Verification items for the finished model (mm, model axes). A direction names the side the tool comes from. Coordinates: 2 decimals unless noted, no trailing zeros. Write each loop counter-clockwise with the first axis right and the second up, starting at its lowest first coordinate (ties: lowest second). Pieces come first, ordered by that corner, then holes. Notation, with made-up numbers: M -17.5,-12.5 L 1.5,-12.5 A15 ccw 1.5,15.5 Z; hole C 1.25,30 d9. An arc over 180 degrees is marked long. Answer in a Markdown table with one row per item.
from build123d import *

# Parameters (mm, degrees)
PAD004_DEPTH    = 29
POCKET001_DEPTH = 5
POCKET002_DEPTH = 5
SKETCH008_R     = 5
POCKET003_DEPTH = 10
SKETCH015_R     = 2
POCKET007_DEPTH = 24.001


with BuildPart() as obj1:
    # Sketch004 → Pad004 (new body)
    with BuildSketch(Plane.XY):
        with BuildLine():
            Line((0, 40), (0, 0))
            Line((0, 0), (160, 0))
            Line((160, 15), (160, 0))
            Line((125, 15), (160, 15))
            ThreePointArc((115, 25), (117.928932, 17.928932), (125, 15))
            Line((115, 42.094566), (115, 25))
            Line((90, 42.094566), (115, 42.094566))
            Line((90, 42.094566), (90, 20))
            ThreePointArc((80, 10), (87.071068, 12.928932), (90, 20))
            Line((30, 10), (80, 10))
            ThreePointArc((10, 30), (15.857864, 15.857864), (30, 10))
            Line((10, 40), (10, 30))
            Line((0, 40), (10, 40))
        make_face()
    extrude(amount=PAD004_DEPTH)

    # Sketch006 (on Face15 of Pad004) → Pocket001 (cut)
    with BuildSketch(Plane.XY.offset(29)):
        Polygon((5, 45), (5, 5), (100, 5), (100, -8.029739), (275.374889, -8.029739), (275.374889, 45), align=None)
    extrude(amount=-POCKET001_DEPTH, mode=Mode.SUBTRACT)

    # Sketch007 (on Face2 of Pocket001) → Pocket002 (cut)
    with BuildSketch(Plane(origin=(0, 0, 0), x_dir=(1, 0, 0), z_dir=(0, 0, -1))):
        Polygon((5, -5), (5, -45), (160, -45), (160, 8.546066), (45, 8.546066), (45, -5), align=None)
    extrude(amount=-POCKET002_DEPTH, mode=Mode.SUBTRACT)

    # Sketch008 (on Face4 of Pocket002) → Pocket003 (cut)
    with BuildSketch(Plane.XY.offset(24)):
        with Locations((110, 10)):
            Circle(SKETCH008_R)
    extrude(amount=-POCKET003_DEPTH, mode=Mode.SUBTRACT)

    # Sketch015 (on Face4 of Pocket003) → Pocket007 (cut, through all)
    with BuildSketch(Plane.XY.offset(24)):
        with Locations((11, 11)):
            Circle(SKETCH015_R)
        with Locations((94, 11)):
            Circle(SKETCH015_R)
        with Locations((94, 36)):
            Circle(SKETCH015_R)
        with Locations((106, 36)):
            Circle(SKETCH015_R)
        with Locations((124, 6)):
            Circle(SKETCH015_R)
        with Locations((154, 6)):
            Circle(SKETCH015_R)
    extrude(amount=-POCKET007_DEPTH, mode=Mode.SUBTRACT)


with BuildPart() as obj1_1:
    # Body004 placement: moved
    add(obj1.part.moved(Location((-250, -150, 0))))


with BuildPart() as obj2:
    # Part__Mirroring001: instance of obj1
    add(obj1_1.part.mirror(Plane(origin=(0, 0, 0), x_dir=(0, -1, 0), z_dir=(1, 0, 0))))


solid = obj2.part
1) Tool access check on faces 1 (the face through (225, -145, 2)), 2 (the face through (234.297, -133.986, 14.367)), 3 (the face through (108, -135, 14)), 4 (the face through (205, -148, 2)), 5 (the face through (140, -140, 14)). Record the directions out of +Z, -Z, +X, -X, +Y, -Y that give a thin tool (end or side, any length) a straight path to the whole face; none if there is none.
Response values:
| item | result |
|---|---|
| face 1 | -Z, -X, +Y |
| face 2 | +Z, -Z, +Y |
| face 3 | +Z, -Z, -X, +Y |
| face 4 | -Z, -X, +Y, -Y |
| face 5 | +Z |
2) Sectioned sample at D-D (x = 162). Record the cut outline in (y, z).
Response values:
| item | result |
|---|---|
| outline | M -150,5 L -136,5 L -136,24 L -145,24 L -145,29 L -150,29 Z |
3) Sectioned sample at B-B (x = 96). Record the cut outline in (y, z), then the cut area to 3 significant figures.
Response values:
| item | result |
|---|---|
| outline | M -150,5 L -146,5 L -146,24 L -150,24 Z; M -142,5 L -135,5 L -135,24 L -142,24 Z |
| area | 209 mm² |
4) Sectioned sample at A-A (y = -114). Record the cut outline in (x, z), then the cut area to 3 significant figures.
Response values:
| item | result |
|---|---|
| outline | M 135,5 L 142,5 L 142,24 L 135,24 Z; M 146,5 L 154,5 L 154,24 L 146,24 Z; M 158,5 L 160,5 L 160,24 L 158,24 Z; M 240,5 L 245,5 L 245,0 L 250,0 L 250,29 L 245,29 L 245,24 L 240,24 Z |
| area | 563 mm² |
5) Sectioned sample at C-C (z = 16.25). Record the cut outline in (x, y), then the cut area to 3 significant figures.
Response values:
| item | result |
|---|---|
| outline | M 90,-150 L 250,-150 L 250,-110 L 240,-110 L 240,-120 A20 cw 220,-140 L 170,-140 A10 cw 160,-130 L 160,-107.91 L 135,-107.91 L 135,-125 A10 cw 125,-135 L 90,-135 Z; hole C 96,-144 d4; hole C 126,-144 d4; hole C 140,-140 d10; hole C 144,-114 d4; hole C 156,-139 d4; hole C 156,-114 d4; hole C 239,-139 d4 |
| area | 2,900 mm² |
6) Depth check by flat-ended pin: pin 1 (8 mm diameter, centred on y = -116, z = 13.5, fed in from -X); pin 2 (4 mm diameter, centred on x = 111.5, y = -136, fed in from -Z); pin 3 (9 mm diameter, centred on x = 140, y = -140, fed in from +Z). Enter the tip coordinate at first touch or a pass-through.
Response values:
| item | result |
|---|---|
| pin 1 | stops at x = 135 |
| pin 2 | stops at z = 5 |
| pin 3 | stops at z = 14 |
7) Thickness scan on L1, parallel to X at y = -114, z = 14.5; L2, parallel to X at y = -144, z = 13.75; L3, parallel to Y at x = 144, z = 13.5. Record the ranges inside material, lowest first. Write a range as [from, to].
Response values:
| item | result |
|---|---|
| L1 | x = [135, 142], [146, 154], [158, 160], [240, 250] |
| L2 | x = [90, 94], [98, 124], [128, 250] |
| L3 | y = [-150, -116], [-112, -107.91] |
